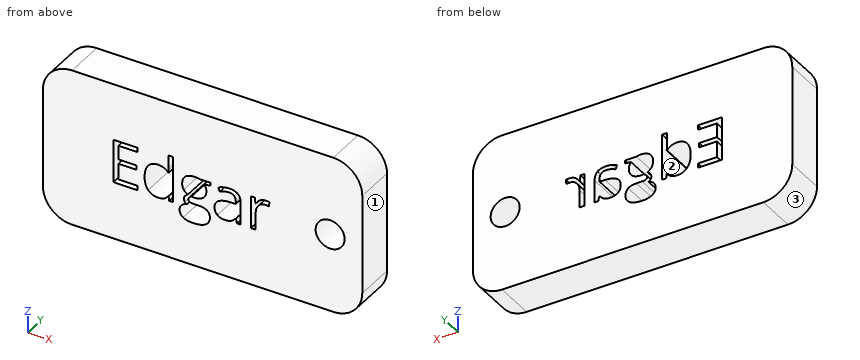
```python
from build123d import *

# Parameters (mm, degrees)
F0_R     = 3.175
F1_DEPTH = 8.89


with BuildPart() as f1:
    # F0 (on Front) → F1 (new body)
    with BuildSketch(Plane.XZ):
        with BuildLine():
            ThreePointArc((-21.9656324044, -6.2401519575), (-20.1057604649, -10.7302800181), (-15.6156324044, -12.5901519575))
            Line((-15.6156324044, -12.5901519575), (41.5343675956, -12.5901519575))
            ThreePointArc((41.5343675956, -12.5901519575), (46.0244956561, -10.7302800181), (47.8843675956, -6.2401519575))
            Line((47.8843675956, -6.2401519575), (47.8843675956, 15.5370884062))
            ThreePointArc((47.8843675956, 15.5370884062), (46.0244956561, 20.0272164667), (41.5343675956, 21.8870884062))
            Line((41.5343675956, 21.8870884062), (-15.6156324044, 21.8870884062))
            ThreePointArc((-15.6156324044, 21.8870884062), (-20.1057604649, 20.0272164667), (-21.9656324044, 15.5370884062))
            Line((-21.9656324044, 15.5370884062), (-21.9656324044, -6.2401519575))
        make_face()
        with BuildLine():
            Line((12.1711680144, 7.1195565384), (14.6323519389, 7.1195565384))
            Line((14.6323519389, 7.1195565384), (14.6323519389, 6.4377420729))
            Line((14.6323519389, 6.4377420729), (13.3144544658, 6.2818393749))
            add(Edge.make_bspline(
                [(13.3144544658, 6.2818393749), (13.4953015954, 6.0552607873), (13.6387320775, 5.6873304202)],
                knots=[0, 0, 0, 1, 1, 1], degree=2))
            add(Edge.make_bspline(
                [(13.6387320775, 5.6873304202), (13.7821625596, 5.3194000531), (13.7821625596, 4.8600067699)],
                knots=[0, 0, 0, 1, 1, 1], degree=2))
            add(Edge.make_bspline(
                [(13.7821625596, 4.8600067699), (13.7821625596, 3.8123406398), (13.0670888518, 3.1887298482)],
                knots=[0, 0, 0, 1, 1, 1], degree=2))
            add(Edge.make_bspline(
                [(13.0670888518, 3.1887298482), (12.352015144, 2.5651190565), (11.1047935606, 2.5651190565)],
                knots=[0, 0, 0, 1, 1, 1], degree=2))
            add(Edge.make_bspline(
                [(11.1047935606, 2.5651190565), (10.7867520569, 2.5651190565), (10.5082059032, 2.6170866224)],
                knots=[0, 0, 0, 1, 1, 1], degree=2))
            add(Edge.make_bspline(
                [(10.5082059032, 2.6170866224), (9.8201553297, 2.2533136606), (9.8201553297, 1.7024574613)],
                knots=[0, 0, 0, 1, 1, 1], degree=2))
            add(Edge.make_bspline(
                [(9.8201553297, 1.7024574613), (9.8201553297, 1.4093603892), (10.0602454845, 1.2700873124)],
                knots=[0, 0, 0, 1, 1, 1], degree=2))
            add(Edge.make_bspline(
                [(10.0602454845, 1.2700873124), (10.3003356393, 1.1308142356), (10.8844510809, 1.1308142356)],
                knots=[0, 0, 0, 1, 1, 1], degree=2))
            Line((10.8844510809, 1.1308142356), (12.1441448801, 1.1308142356))
            add(Edge.make_bspline(
                [(12.1441448801, 1.1308142356), (13.30198225, 1.1308142356), (13.9214356364, 0.6433584668)],
                knots=[0, 0, 0, 1, 1, 1], degree=2))
            add(Edge.make_bspline(
                [(13.9214356364, 0.6433584668), (14.5408890228, 0.1559026979), (14.5408890228, -0.7732773817)],
                knots=[0, 0, 0, 1, 1, 1], degree=2))
            add(Edge.make_bspline(
                [(14.5408890228, -0.7732773817), (14.5408890228, -1.9560591833), (13.5930006194, -2.576551921)],
                knots=[0, 0, 0, 1, 1, 1], degree=2))
            add(Edge.make_bspline(
                [(13.5930006194, -2.576551921), (12.6451122161, -3.1970446587), (10.826247407, -3.1970446587)],
                knots=[0, 0, 0, 1, 1, 1], degree=2))
            add(Edge.make_bspline(
                [(10.826247407, -3.1970446587), (9.4293592336, -3.1970446587), (8.672711473, -2.677368999)],
                knots=[0, 0, 0, 1, 1, 1], degree=2))
            add(Edge.make_bspline(
                [(8.672711473, -2.677368999), (7.9160637125, -2.1576933392), (7.9160637125, -1.2077262332)],
                knots=[0, 0, 0, 1, 1, 1], degree=2))
            add(Edge.make_bspline(
                [(7.9160637125, -1.2077262332), (7.9160637125, -0.5591710099), (8.3318042402, -0.0841874569)],
                knots=[0, 0, 0, 1, 1, 1], degree=2))
            add(Edge.make_bspline(
                [(8.3318042402, -0.0841874569), (8.747544768, 0.3907960961), (9.5000351233, 0.5591710099)],
                knots=[0, 0, 0, 1, 1, 1], degree=2))
            add(Edge.make_bspline(
                [(9.5000351233, 0.5591710099), (9.2277250776, 0.6818144656), (9.0427205428, 0.9416522954)],
                knots=[0, 0, 0, 1, 1, 1], degree=2))
            add(Edge.make_bspline(
                [(9.0427205428, 0.9416522954), (8.8577160079, 1.2014901253), (8.8577160079, 1.5465547634)],
                knots=[0, 0, 0, 1, 1, 1], degree=2))
            add(Edge.make_bspline(
                [(8.8577160079, 1.5465547634), (8.8577160079, 1.9352721569), (9.0655862718, 2.228369229)],
                knots=[0, 0, 0, 1, 1, 1], degree=2))
            add(Edge.make_bspline(
                [(9.0655862718, 2.228369229), (9.2734565357, 2.5214663011), (9.7224563057, 2.7937763468)],
                knots=[0, 0, 0, 1, 1, 1], degree=2))
            add(Edge.make_bspline(
                [(9.7224563057, 2.7937763468), (9.1695214037, 3.0203549344), (8.822378063, 3.5660143771)],
                knots=[0, 0, 0, 1, 1, 1], degree=2))
            add(Edge.make_bspline(
                [(8.822378063, 3.5660143771), (8.4752347223, 4.1116738199), (8.4752347223, 4.8142753118)],
                knots=[0, 0, 0, 1, 1, 1], degree=2))
            add(Edge.make_bspline(
                [(8.4752347223, 4.8142753118), (8.4752347223, 5.9825061949), (9.176796863, 6.6165104998)],
                knots=[0, 0, 0, 1, 1, 1], degree=2))
            add(Edge.make_bspline(
                [(9.176796863, 6.6165104998), (9.8783590036, 7.2505148047), (11.1629972345, 7.2505148047)],
                knots=[0, 0, 0, 1, 1, 1], degree=2))
            add(Edge.make_bspline(
                [(11.1629972345, 7.2505148047), (11.7221682444, 7.2505148047), (12.1711680144, 7.1195565384)],
                knots=[0, 0, 0, 1, 1, 1], degree=2))
        make_face(mode=Mode.SUBTRACT)
        with BuildLine():
            Line((21.2717281678, 0), (20.4714276518, 0))
            Line((20.4714276518, 0), (20.2573212799, 1.0144068878))
            Line((20.2573212799, 1.0144068878), (20.205353714, 1.0144068878))
            add(Edge.make_bspline(
                [(20.205353714, 1.0144068878), (19.6732058384, 0.3450646381), (19.1441760168, 0.1070531859)],
                knots=[0, 0, 0, 1, 1, 1], degree=2))
            add(Edge.make_bspline(
                [(19.1441760168, 0.1070531859), (18.6151461952, -0.1309582663), (17.8210817871, -0.1309582663)],
                knots=[0, 0, 0, 1, 1, 1], degree=2))
            add(Edge.make_bspline(
                [(17.8210817871, -0.1309582663), (16.7630221439, -0.1309582663), (16.1622770812, 0.4157405278)],
                knots=[0, 0, 0, 1, 1, 1], degree=2))
            add(Edge.make_bspline(
                [(16.1622770812, 0.4157405278), (15.5615320185, 0.9624393218), (15.5615320185, 1.9685313991)],
                knots=[0, 0, 0, 1, 1, 1], degree=2))
            add(Edge.make_bspline(
                [(15.5615320185, 1.9685313991), (15.5615320185, 4.1241460357), (19.0100996966, 4.2280811676)],
                knots=[0, 0, 0, 1, 1, 1], degree=2))
            Line((19.0100996966, 4.2280811676), (20.2178259298, 4.2675765178))
            Line((20.2178259298, 4.2675765178), (20.2178259298, 4.7103401799))
            add(Edge.make_bspline(
                [(20.2178259298, 4.7103401799), (20.2178259298, 5.5480573434), (19.8582103733, 5.9471682501)],
                knots=[0, 0, 0, 1, 1, 1], degree=2))
            add(Edge.make_bspline(
                [(19.8582103733, 5.9471682501), (19.4985948167, 6.3462791567), (18.7045304086, 6.3462791567)],
                knots=[0, 0, 0, 1, 1, 1], degree=2))
            add(Edge.make_bspline(
                [(18.7045304086, 6.3462791567), (17.8148456792, 6.3462791567), (16.6923462541, 5.8016590653)],
                knots=[0, 0, 0, 1, 1, 1], degree=2))
            Line((16.6923462541, 5.8016590653), (16.3597538319, 6.626904013))
            add(Edge.make_bspline(
                [(16.3597538319, 6.626904013), (16.8856655996, 6.9116862745), (17.5123944452, 7.0738250804)],
                knots=[0, 0, 0, 1, 1, 1], degree=2))
            add(Edge.make_bspline(
                [(17.5123944452, 7.0738250804), (18.1391232908, 7.2359638862), (18.7710488931, 7.2359638862)],
                knots=[0, 0, 0, 1, 1, 1], degree=2))
            add(Edge.make_bspline(
                [(18.7710488931, 7.2359638862), (20.0432149081, 7.2359638862), (20.6574715379, 6.6715961197)],
                knots=[0, 0, 0, 1, 1, 1], degree=2))
            add(Edge.make_bspline(
                [(20.6574715379, 6.6715961197), (21.2717281678, 6.1072283533), (21.2717281678, 4.8600067699)],
                knots=[0, 0, 0, 1, 1, 1], degree=2))
            Line((21.2717281678, 4.8600067699), (21.2717281678, 0))
        make_face(mode=Mode.SUBTRACT)
        with BuildLine():
            add(Edge.make_bspline(
                [(25.5122815512, 6.8732302757), (26.0714525611, 7.2505148047), (26.7407948108, 7.2505148047)],
                knots=[0, 0, 0, 1, 1, 1], degree=2))
            add(Edge.make_bspline(
                [(26.7407948108, 7.2505148047), (27.2147390125, 7.2505148047), (27.5909841902, 7.1715241044)],
                knots=[0, 0, 0, 1, 1, 1], degree=2))
            Line((27.5909841902, 7.1715241044), (27.4413176002, 6.1716681351))
            add(Edge.make_bspline(
                [(27.4413176002, 6.1716681351), (27.0006326407, 6.2693671591), (26.6618041106, 6.2693671591)],
                knots=[0, 0, 0, 1, 1, 1], degree=2))
            add(Edge.make_bspline(
                [(26.6618041106, 6.2693671591), (25.7970638128, 6.2693671591), (25.1838465343, 5.5678050184)],
                knots=[0, 0, 0, 1, 1, 1], degree=2))
            add(Edge.make_bspline(
                [(25.1838465343, 5.5678050184), (24.5706292558, 4.8662428778), (24.5706292558, 3.8206554504)],
                knots=[0, 0, 0, 1, 1, 1], degree=2))
            Line((24.5706292558, 3.8206554504), (24.5706292558, 0))
            Line((24.5706292558, 0), (23.4917825862, 0))
            Line((23.4917825862, 0), (23.4917825862, 7.1195565384))
            Line((23.4917825862, 7.1195565384), (24.3814673156, 7.1195565384))
            Line((24.3814673156, 7.1195565384), (24.506189474, 5.8016590653))
            Line((24.506189474, 5.8016590653), (24.5581570399, 5.8016590653))
            add(Edge.make_bspline(
                [(24.5581570399, 5.8016590653), (24.9531105413, 6.4959457467), (25.5122815512, 6.8732302757)],
                knots=[0, 0, 0, 1, 1, 1], degree=2))
        make_face(mode=Mode.SUBTRACT)
        with Locations((40.8501774073, 4.5076054521)):
            Circle(F0_R, mode=Mode.SUBTRACT)
        Polygon((-1.2884315729, 0.9873837535), (-1.2884315729, 0), (-6.5828871943, 0), (-6.5828871943, 9.4975923574), (-1.2884315729, 9.4975923574), (-1.2884315729, 8.5164447118), (-5.479096093, 8.5164447118), (-5.479096093, 5.4565944273), (-1.5420332948, 5.4565944273), (-1.5420332948, 4.4816828896), (-5.479096093, 4.4816828896), (-5.479096093, 0.9873837535), align=None, mode=Mode.SUBTRACT)
        with BuildLine():
            Line((5.6419630254, 0), (5.4985325433, 0.9541245113))
            Line((5.4985325433, 0.9541245113), (5.4403288695, 0.9541245113))
            add(Edge.make_bspline(
                [(5.4403288695, 0.9541245113), (4.6940746221, -0.1309582663), (3.2057235326, -0.1309582663)],
                knots=[0, 0, 0, 1, 1, 1], degree=2))
            add(Edge.make_bspline(
                [(3.2057235326, -0.1309582663), (1.8088353592, -0.1309582663), (1.0324399235, 0.8242055963)],
                knots=[0, 0, 0, 1, 1, 1], degree=2))
            add(Edge.make_bspline(
                [(1.0324399235, 0.8242055963), (0.2560444879, 1.7793694589), (0.2560444879, 3.5400305941)],
                knots=[0, 0, 0, 1, 1, 1], degree=2))
            add(Edge.make_bspline(
                [(0.2560444879, 3.5400305941), (0.2560444879, 5.3006917293), (1.0355579775, 6.275603267)],
                knots=[0, 0, 0, 1, 1, 1], degree=2))
            add(Edge.make_bspline(
                [(1.0355579775, 6.275603267), (1.8150714671, 7.2505148047), (3.2057235326, 7.2505148047)],
                knots=[0, 0, 0, 1, 1, 1], degree=2))
            add(Edge.make_bspline(
                [(3.2057235326, 7.2505148047), (4.6545792719, 7.2505148047), (5.4278566536, 6.1966125667)],
                knots=[0, 0, 0, 1, 1, 1], degree=2))
            Line((5.4278566536, 6.1966125667), (5.5130834618, 6.1966125667))
            Line((5.5130834618, 6.1966125667), (5.4673520038, 6.7100521186))
            Line((5.4673520038, 6.7100521186), (5.4403288695, 7.2110194545))
            Line((5.4403288695, 7.2110194545), (5.4403288695, 10.1087309332))
            Line((5.4403288695, 10.1087309332), (6.5191755391, 10.1087309332))
            Line((6.5191755391, 10.1087309332), (6.5191755391, 0))
            Line((6.5191755391, 0), (5.6419630254, 0))
        make_face(mode=Mode.SUBTRACT)
    extrude(amount=F1_DEPTH)


solid = f1.part
```
For this review, take the finished solid that the model builds, in its own axes (mm). Face numbers are marked on the shaded views. Round coordinates to 2 decimals unless told otherwise and drop trailing zeros. Use one line per item in the form item = value.
Q1. Clearance check with flat-ended pins moving along their axes: pin 1 Ø5 at (x, z) = (40.85, 4.51) entering from +Y; pin 2 Ø12 at (x, z) = (13.5, -8) entering from +Y. State where each tip first meets the part, or that it passes through.
Resolved:
pin_1 = through
pin_2 = 0
Q2. To check wall thickness, follow probe 1 along Z at (x, y) = (18, -2.75); probe 2 along X at (y, z) = (-1, 8); probe 3 along Z at (x, y) = (17.5, -8). State the ranges of each line that lie inside material, in increasing order. Write a range as from..to.
Resolved:
probe_1 = -12.59..-0.13, 4.14..6.27, 7.18..21.89
probe_2 = -21.97..-6.58, -5.48..5.44, 6.52..47.88
probe_3 = -12.59..-0.12, 4.05..6.13, 7.07..21.89
Q3. The part is to be moulded in two halves that separate along Z. For the marked faces 1, 2 and 3, say which applies: released by +Z, released by -Z, zero draft, split by the parting line, or undercut.
Resolved:
face_1 = zero draft
face_2 = undercut
face_3 = released by -Z
Q4. Consider section A-A (y = -4). State how many separate pieces and enclosed holes the cut face has, then the cut area to 3 significant figures.
Resolved:
separate_pieces = 1
enclosed_holes = 6
area = 2,190 mm²
